Geometry check sheet. Reference: the model listing, model coordinates, mm. Coordinates: 2 decimals unless noted, no trailing zeros. Write each loop counter-clockwise with the first axis right and the second up, starting at its lowest first coordinate (ties: lowest second). Pieces come first, ordered by that corner, then holes. Notation, with made-up numbers: (63.25, 2.5) -> (99.25, 2.5) arc R17 cw to (99.25, 22.5) -> close; hole circle Ø6 at (-12, -38). An arc over 180 degrees is marked (long way). One line per question, with ' | ' between items.
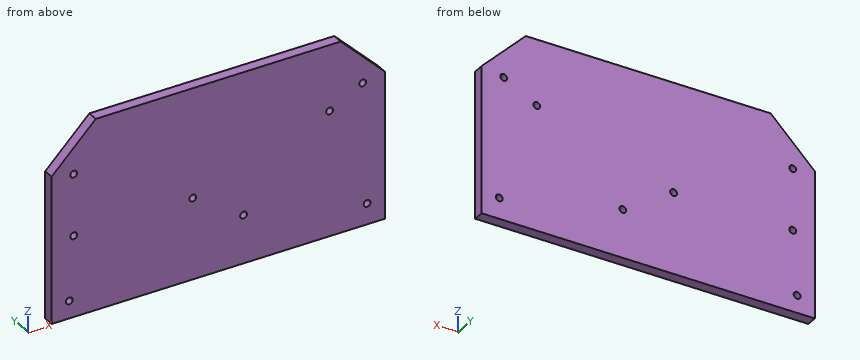
```python
from build123d import *

# Parameters (mm, degrees)
F0_W     = 151
F0_H     = 87
F1_DEPTH = 4.8
F2_R     = 1.55
F3_DEPTH = 4.8
F4_DEPTH = 4.8
F5_SIZE  = 20
F6_SIZE  = 20


with BuildPart() as f1:
    # F0 (on Front) → F1 (new body)
    with BuildSketch(Plane.XZ):
        Rectangle(F0_W, F0_H)
    extrude(amount=F1_DEPTH)

    # F2 (on face) → F3 (cut)
    with BuildSketch(Plane.XZ.offset(4.8)):
        with Locations((-65.5, -6.5)):
            Circle(F2_R)
    extrude(amount=-F3_DEPTH, mode=Mode.SUBTRACT)

    # F2 (on face) → F4 (cut)
    with BuildSketch(Plane.XZ.offset(4.8)):
        with Locations((-65.5, 21.5)):
            Circle(F2_R)
        with Locations((65.5, 21.5)):
            Circle(F2_R)
        with Locations((-67.5, -35.5)):
            Circle(F2_R)
        with Locations((67.5, -33.95)):
            Circle(F2_R)
        with Locations((50.5, 13.5)):
            Circle(F2_R)
        with Locations((11.5, -21.5)):
            Circle(F2_R)
        with Locations((-65.5, -6.5)):
            Circle(F2_R)
        with Locations((-11.5, -6.5)):
            Circle(F2_R)
    extrude(amount=-F4_DEPTH, mode=Mode.SUBTRACT)

    # F5
    f5_edges = [f1.edges().sort_by_distance(p)[0] for p in [
        (-75.5, -2.4, 43.5),
    ]]
    chamfer(f5_edges, length=F5_SIZE)

    # F6
    f6_edges = [f1.edges().sort_by_distance(p)[0] for p in [
        (75.5, -2.4, 43.5),
    ]]
    chamfer(f6_edges, length=F6_SIZE)


solid = f1.part
```
(1) Depth check by flat-ended pin: P1, Ø1.9, axis at x = -11.5, z = -6.5, coming from the +Y side. Enter the tip coordinate at first touch or a pass-through.
Answers below:
P1: passes through
(2) Cross-section at A-A (x = 50.5). Record the cut outline in (y, z).
Answers below:
outline: (-4.8, -43.5) -> (0, -43.5) -> (0, 11.95) -> (-4.8, 11.95) -> close; (-4.8, 15.05) -> (0, 15.05) -> (0, 43.5) -> (-4.8, 43.5) -> close
(3) Cross-section at C-C (z = -6.5). Record the cut outline in (x, y), plus the area to 3 significant figures.
Answers below:
outline: (-75.5, -4.8) -> (-67.05, -4.8) -> (-67.05, 0) -> (-75.5, 0) -> close; (-63.95, -4.8) -> (-13.05, -4.8) -> (-13.05, 0) -> (-63.95, 0) -> close; (-9.95, -4.8) -> (75.5, -4.8) -> (75.5, 0) -> (-9.95, 0) -> close | area: 695 mm²
(4) Material ranges on line 1 (Z direction, x = 11.5, y = -1.9); line 2 (Z direction, x = -65.5, y = -2.6); line 3 (Z direction, x = 50.5, y = -2.75), recorded low to high.
Answers below:
line 1: z = -43.5 to -23.05, -19.95 to 43.5 | line 2: z = -43.5 to -8.05, -4.95 to 19.95, 23.05 to 33.5 | line 3: z = -43.5 to 11.95, 15.05 to 43.5
(5) Cross-section at D-D (y = -0.9). Count the separate pieces of the cut face and the enclosed holes in it, plus the area to 3 significant figures.
Answers below:
separate pieces: 1 | enclosed holes: 8 | area: 12,700 mm²
(6) Cross-section at B-B (z = 13.5). Record the cut outline in (x, y).
Answers below:
outline: (-75.5, -4.8) -> (48.95, -4.8) -> (48.95, 0) -> (-75.5, 0) -> close; (52.05, -4.8) -> (75.5, -4.8) -> (75.5, 0) -> (52.05, 0) -> close
